Geometry: final body of the model. Coordinates: model frame, mm. Give positions to 0.01 mm unless a question says otherwise; leave off trailing zeros. Write each loop counter-clockwise with the first axis right and the second up, starting at its lowest first coordinate (ties: lowest second). Pieces come first, ordered by that corner, then holes. Notation, with made-up numbers: M -30.75,73.25 L -3.75,73.25 A19 cw -3.75,107.25 Z; hole C 17,10.25 d3. An arc over 180 degrees is marked long. Use a Markdown table: item, result. Add a question column.
1) Line query: line 1 (Y direction, x = 0, z = 0.7); line 2 (X direction, y = -0.5, z = 1.4); line 3 (Y direction, x = -4.5, z = 0.4). Output: solid intervals per line, ascending.
2) Section D-D on x = 52. Return the cut outline in (y, z).
3) Draft query along X for faces 1 (the flat face through (-1, 15, 1.588)), 2 (the flat face through (-27.385, -34.731, 0.805)). Return one class per face: +X half, -X half, draft (parallel to the pull), parting line (faces both ways), or undercut.
4) Section B-B on y = 0. Return the cut outline in (x, z).
5) Section A-A on x = 0. Return the cut outline in (y, z), then the cut area to 3 significant figures.
6) Section C-C on z = 0.3. State how many separate pieces and enclosed holes the cut face has, then the cut area to 3 significant figures.
7) Pin query (flat end, axial travel): pin 1 (23 mm diameter, centred on x = 0, y = 0, fed in from +Z); pin 2 (4 mm diameter, centred on x = -12, y = 25.5, fed in from -Z); pin 3 (0.8 mm diameter, centred on x = 44.5, z = 0.5, fed in from +Y); pin 4 (0.8 mm diameter, centred on y = 2.5, z = 1, fed in from +X). Return the tip coordinate at first contact, or that it passes through.
```python
from build123d import *

# Parameters (mm, degrees)
F0_R            = 63.5
F0_R_2          = 14.4272
F1_DEPTH        = 1.5875
F2_W            = 12.7
F2_H            = 6.35
F3_DEPTH        = 1.5885
F3_COPIES_COUNT = 12
F4_R            = 2.4892
F5_DEPTH        = 1.5885
F5_COPIES_COUNT = 6


# Not quite as in the source:
# - a pattern or mirror of a feature is missing from the dataset's text; its kind, count and spacing are read off the source's solid


with BuildPart() as f1:
    # F0 (on Top) → F1 (new body)
    with BuildSketch(Plane.XY):
        Circle(F0_R)
        Circle(F0_R_2, mode=Mode.SUBTRACT)
    extrude(amount=F1_DEPTH)

    # F2 (on face) → F3 (cut, through all)
    with BuildSketch(Plane.XY.offset(1.5875)):
        with Locations((0, 43.815)):
            Rectangle(F2_W, F2_H)
    f3 = extrude(amount=-F3_DEPTH, mode=Mode.SUBTRACT)

    # F3_copies: F3 ×12 about axis
    f3_copies_axis = Axis((0, 0, 0), (0, 0, 1))
    for i in range(1, F3_COPIES_COUNT):
        add(f3.rotate(f3_copies_axis, i * 360 / F3_COPIES_COUNT), mode=Mode.SUBTRACT)

    # F4 (on face) → F5 (cut, through all)
    with BuildSketch(Plane.XY.offset(1.5875)):
        with Locations((0, 23.8125)):
            Circle(F4_R)
    f5 = extrude(amount=-F5_DEPTH, mode=Mode.SUBTRACT)

    # F5_copies: F5 ×6 about axis
    f5_copies_axis = Axis((0, 0, 0), (0, 0, 1))
    for i in range(1, F5_COPIES_COUNT):
        add(f5.rotate(f5_copies_axis, i * 360 / F5_COPIES_COUNT), mode=Mode.SUBTRACT)


solid = f1.part
```
Found:
| question | item | result |
|---|---|---|
| 1 | line 1 | -63.5 to -46.99, -40.64 to -26.3, -21.32 to -14.43, 14.43 to 21.32, 26.3 to 40.64, 46.99 to 63.5 |
| 1 | line 2 | -63.5 to -46.99, -40.64 to -14.42, 14.42 to 40.64, 46.99 to 63.5 |
| 1 | line 3 | -63.34 to -46.99, -40.64 to -13.71, 13.71 to 40.64, 46.99 to 63.34 |
| 2 | outline | M -36.45,0 L 36.45,0 L 36.45,1.59 L -36.45,1.59 Z |
| 3 | face 1 | draft |
| 3 | face 2 | undercut |
| 4 | outline | M -63.5,0 L -46.99,0 L -46.99,1.59 L -63.5,1.59 Z; M -40.64,0 L -14.43,0 L -14.43,1.59 L -40.64,1.59 Z; M 14.43,0 L 40.64,0 L 40.64,1.59 L 14.43,1.59 Z; M 46.99,0 L 63.5,0 L 63.5,1.59 L 46.99,1.59 Z |
| 5 | outline | M -63.5,0 L -46.99,0 L -46.99,1.59 L -63.5,1.59 Z; M -40.64,0 L -26.3,0 L -26.3,1.59 L -40.64,1.59 Z; M -21.32,0 L -14.43,0 L -14.43,1.59 L -21.32,1.59 Z; M 14.43,0 L 21.32,0 L 21.32,1.59 L 14.43,1.59 Z; M 26.3,0 L 40.64,0 L 40.64,1.59 L 26.3,1.59 Z; M 46.99,0 L 63.5,0 L 63.5,1.59 L 46.99,1.59 Z |
| 5 | area | 120 mm² |
| 6 | separate pieces | 1 |
| 6 | enclosed holes | 19 |
| 6 | area | 10,900 mm² |
| 7 | pin 1 | through |
| 7 | pin 2 | z = 0 |
| 7 | pin 3 | y = 45.69 |
| 7 | pin 4 | x = 63.47 |
